Design review of the part built by this model. Coordinates are the model's own, in mm. Face numbers are marked on the shaded views. A direction names the side the tool comes from. Coordinates: 2 decimals unless noted, no trailing zeros. Loops run counter-clockwise (first coordinate to the right, second up) from the corner with the lowest first, then second, coordinate; pieces in that order, holes last.
Q1. Wall thickness on probe 1 along X at (y, z) = (3.25, 1.35); probe 2 along X at (y, z) = (6, 1.85); probe 3 along Y at (x, z) = (4, 1.9): over which ranges is each line inside the solid? List them lowest first.
Q2. Add section A-A on z = 1.85. Give the boundary of the cut face in (x, y).
Q3. Machinability: for the marked faces 5 and 6, which of the approach directions +Z, -Z, +X, -X, +Y, -Y give a long, thin tool a straight path to every point of the face, cutting with its end or side? Answer none if there is none.
Q4. Add section C-C on y = 8.75. Give the boundary of the cut face in (x, z), and give its area (3 significant figures).
Q5. Add section B-B on x = 1.25. Give the boundary of the cut face in (y, z).
Q6. Draft analysis for pull direction X (two halves, no side actions). For the marked faces 1, 2, 3 and 4, state which applies: released by +X, released by -X, zero draft, split by the parting line, or undercut.
Q7. For P1, Ø2.5, axis at x = 3.5, y = 9, coming from the +Z side; P2, Ø2.5, axis at x = 5, y = 7, coming from the +Z side, all flat-tipped, find the tip position at first contact; note any pin that passes through.
Autodesk Inventor part; units mm, degrees
ref_plane "YZ Plane" through (0, 0, 0) normal (1, 0, 0) x (0, 1, 0)
ref_plane "XZ Plane" through (0, 0, 0) normal (0, 1, 0) x (-1, 0, 0)
ref_plane "XY Plane" through (0, 0, 0) normal (0, 0, 1) x (1, 0, 0)
sketch "Sketch1" plane through (0, 0, 0) normal (0, 0, 1) x (1, 0, 0)
  line L0 (0, 0) -> (10, 0)
  line L1 (10, 0) -> (10, 15)
  line L2 (10, 15) -> (0, 15)
  line L3 (0, 15) -> (0, 0)
  line L4 (9, 1) -> (1, 1)
  line L5 (1, 1) -> (1, 14)
  line L6 (1, 14) -> (9, 14)
  line L7 (9, 14) -> (9, 1)
  dimension "d0" = 10
  dimension "d1" = 15
  dimension "d2" = 1
extrude "Extrusion1" add sketch "Sketch1" along normal blind 1 contours L4 L5 L6 L7
sketch "Sketch2" plane through (0, 0, 0) normal (0, 0, -1) x (-1, 0, 0)
  line L0 (-1, 1) -> (-9, 1)
  line L1 (-9, 14) -> (-1, 14)
  line L2 (-9, 1) -> (-1, 1)
  line L3 (-1, 1) -> (-1, 14)
  line L4 (-1, 14) -> (-9, 14)
  line L5 (-9, 14) -> (-9, 1)
  point P0 (0, 0)
extrude "Extrusion2" add sketch "Sketch1" along normal blind 2
sketch "Sketch3" plane through (0, 0, 1) normal (0, 0, 1) x (1, 0, 0)
  line L0 (9, 1) -> (1, 1)
  line L1 (3, 1) -> (7, 1)
  line L2 (7, 1) -> (7, 5)
  line L3 (7, 5) -> (3, 5)
  line L4 (3, 5) -> (3, 1)
  line L5 (9, 14) -> (9, 1)
  line L6 (3, 5) -> (7, 5)
  line L7 (7, 5) -> (5, 8)
  line L8 (5, 8) -> (3, 5)
  line L9 (6.1824, 6.2265) -> (6.1824, 7.2265)
  line L10 (6.1824, 7.2265) -> (6.6824, 7.2265)
  line L11 (6.6824, 7.2265) -> (6.6824, 5.4765)
  point P0 (0, 0)
  dimension "d7" = 4
  dimension "d8" = 4
  dimension "d9" = 2
  dimension "d10" = 3
  dimension "d11" = 1
  dimension "d12" = 0.5
extrude "Extrusion3" add sketch "Sketch3" along normal blind 0.5 contours L0 L4 L3 L2
extrude "Extrusion4" add sketch "Sketch3" along normal blind 0.499 contours L3 L8 L7
extrude "Extrusion5" add sketch "Sketch3" along normal blind 0.498 contours L7 L9 L10 L11
properties part number "Painting"
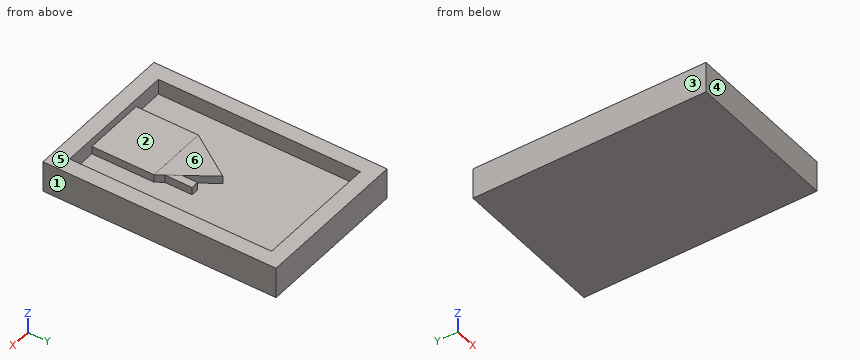
Entries:
1. probe 1: x = 0 to 1, 3 to 7, 9 to 10
1. probe 2: x = 0 to 1, 9 to 10
1. probe 3: y = 0 to 1, 14 to 15
2. outline: (0, 0) - (10, 0) - (10, 15) - (0, 15) - close; hole (1, 1) - (9, 1) - (9, 14) - (1, 14) - close
3. face 5: +Z, +X, -X, +Y, -Y
3. face 6: +Z
4. outline: (0, 0) - (10, 0) - (10, 2) - (9, 2) - (9, 1) - (1, 1) - (1, 2) - (0, 2) - close
4. area: 12.0 mm2
5. outline: (0, 0) - (15, 0) - (15, 2) - (14, 2) - (14, 1) - (1, 1) - (1, 2) - (0, 2) - close
6. face 1: released by +X
6. face 2: undercut
6. face 3: released by -X
6. face 4: zero draft
7. P1: stops at z = 1
7. P2: stops at z = 1.5
